from build123d import *

# Parameters (mm, degrees)
SKETCH018_W  = 26
SKETCH018_H  = 20
SKETCH018_R  = 1.1
PAD011_DEPTH = 1.6
SKETCH019_W  = 17.6
SKETCH019_H  = 18
PAD012_DEPTH = 0.8
CHAMFER_SIZE = 0.6


with BuildPart() as part:
    # Sketch018 → Pad011 (new body)
    with BuildSketch(Plane.XY):
        Rectangle(SKETCH018_W, SKETCH018_H)
        with Locations((-11, -2)):
            Circle(SKETCH018_R, mode=Mode.SUBTRACT)
        with Locations((11, -2)):
            Circle(SKETCH018_R, mode=Mode.SUBTRACT)
    extrude(amount=PAD011_DEPTH)

    # Sketch019 (on Face7 of Pad011) → Pad012 (join)
    with BuildSketch(Plane(origin=(0, 0, 0), x_dir=(1, 0, 0), z_dir=(0, 0, -1))):
        Rectangle(SKETCH019_W, SKETCH019_H)
    extrude(amount=PAD012_DEPTH)

    # Chamfer
    chamfer_edges = [part.edges().sort_by_distance(p)[0] for p in [
        (0, -10, 1.6),
        (0, 10, 1.6),
    ]]
    chamfer(chamfer_edges, length=CHAMFER_SIZE)


with BuildPart() as part_1:
    # Body005 placement: moved
    add(part.part.moved(Location((0, -10, 6))))


solid = part_1.part
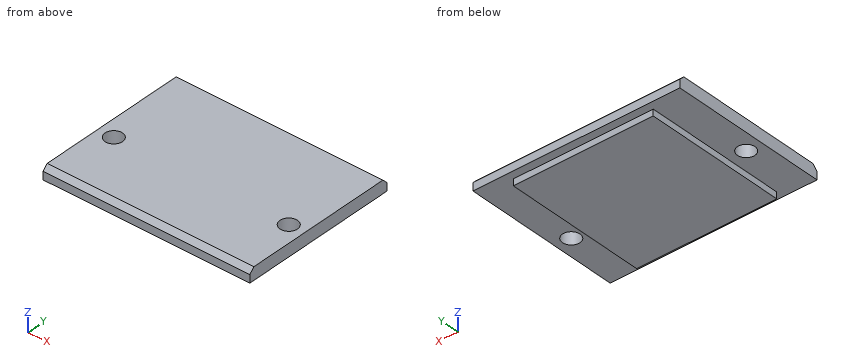
Build history of the part. All positions in model axes, mm. Round coordinates to 2 decimals unless told otherwise and drop trailing zeros. Write each loop counter-clockwise with the first axis right and the second up, starting at its lowest first coordinate (ties: lowest second). Pieces come first, ordered by that corner, then holes. Notation, with made-up numbers: (38.25, 31) - (80.25, 31) arc R21 ccw to (80.25, 66) - close; hole circle Ø9 at (24, 48.5). An arc over 180 degrees is marked (long way). One line per question, with ' | ' between items.
1. Drill centre lines: line 1 along Y through (x, z) = (11, 6.85); line 2 along Z through (x, y) = (11.25, -18.25); line 3 along Y through (x, z) = (-2.5, 5.9). Where is each one in solid material? Low to high. Write a range as from..to.
Results are:
line 1: -20..-13.1, -10.9..0 | line 2: 6..7.6 | line 3: -19..-1
2. Band-saw the part on A-A, the plane x = 11. Write the cut outline in (y, z), and give its area (3 significant figures).
Results are:
outline: (-20, 6) - (-13.1, 6) - (-13.1, 7.6) - (-19.4, 7.6) - (-20, 7) - close; (-10.9, 6) - (0, 6) - (0, 7) - (-0.6, 7.6) - (-10.9, 7.6) - close | area: 28.1 mm^2
3. Band-saw the part on C-C, the plane x = -2.75. Write the cut outline in (y, z).
Results are:
outline: (-20, 6) - (-19, 6) - (-19, 5.2) - (-1, 5.2) - (-1, 6) - (0, 6) - (0, 7) - (-0.6, 7.6) - (-19.4, 7.6) - (-20, 7) - close
4. Band-saw the part on B-B, the plane y = -12. Write the cut outline in (x, z), and give its area (3 significant figures).
Results are:
outline: (-13, 6) - (-12.1, 6) - (-12.1, 7.6) - (-13, 7.6) - close; (-9.9, 6) - (-8.8, 6) - (-8.8, 5.2) - (8.8, 5.2) - (8.8, 6) - (9.9, 6) - (9.9, 7.6) - (-9.9, 7.6) - close; (12.1, 6) - (13, 6) - (13, 7.6) - (12.1, 7.6) - close | area: 48.6 mm^2
5. Drop flat-ended pins along their axis: pin 1 Ø3 at (x, y) = (-11, -12) entering from -Z; pin 2 Ø0.6 at (y, z) = (-9.5, 5.5) entering from +X. Give the stop position or say it passes through.
Results are:
pin 1: z = 6 | pin 2: x = 8.8
6. Band-saw the part on D-D, the plane y = -5.5. Write the cut outline in (x, z), and give its area (3 significant figures).
Results are:
outline: (-13, 6) - (-8.8, 6) - (-8.8, 5.2) - (8.8, 5.2) - (8.8, 6) - (13, 6) - (13, 7.6) - (-13, 7.6) - close | area: 55.7 mm^2
